Work out the finished part from the listing and answer in its coordinate system (mm). Face numbers are marked on the shaded views. A direction names the side the tool comes from. Give positions to 0.01 mm unless a question says otherwise; leave off trailing zeros. Loops run counter-clockwise (first coordinate to the right, second up) from the corner with the lowest first, then second, coordinate; pieces in that order, holes last. Notation, with made-up numbers: M 13.5,16.25 L 35.5,16.25 A11 cw 35.5,31.25 Z; hole C 83.5,-24 d10. An arc over 180 degrees is marked long. Write item = value, one per line. Start each with the question number.
1. Section B-B on z = 1.5 is taken. Determine the outline of the cut face in (x, y), plus the area to 3 significant figures.
2. Flat-ended cylindrical pins translate along their axes: pin 1 Ø6 at (x, z) = (9, 12) entering from +Y; pin 2 Ø4 at (x, y) = (0, -26.5) entering from -Z; pin 3 Ø5 at (y, z) = (18, 7) entering from -X; pin 4 Ø6 at (x, z) = (13, 8) entering from -Y. Find the tip coordinate at first contact, or state that the pin passes through.
3. For the marked faces 5, 6 and 7, determine the directions among +Z, -Z, +X, -X, +Y, -Y from which every point of the face is accessible in a straight line to the end or side of a thin tool.
4. Section C-C on y = -4 is taken. Determine the outline of the cut face in (x, z).
5. Section A-A on x = 0 is taken. Determine the outline of the cut face in (y, z), plus the area to 3 significant figures.
6. Section D-D on z = 9.5 is taken. Determine the outline of the cut face in (x, y), plus the area to 3 significant figures.
7. Consider L1, parallel to Y at x = 0, z = 4.25; L2, parallel to Z at x = 13, y = -1; L3, parallel to X at y = -26.5, z = 3.75. Determine where each line is inside the solid, lowest interval first. Write a range as [from, to].
8. The mould has two halves that part along Y. Classify the marked faces 1, 2, 3 and 4: released by +Y, released by -Y, zero draft, split by the parting line, or undercut.
```python
from build123d import *

# Parameters (mm, degrees)
SKETCH_1_R          = 21
EXTRUDE_2_DEPTH     = 6.5
EXTRUDE_4_DEPTH     = 6.5
SKETCH_3_R          = 9.5
SKETCH_3_R_2        = 3.5
CUT_EXTRUDE_1_DEPTH = 41.068691019


with BuildPart() as part:
    # 草图1 → 凸台-拉伸2 (new body)
    with BuildSketch(Plane.XY):
        with Locations(Location((0, 0, 0), (0, 0, 180))):
            Circle(SKETCH_1_R)
    extrude(amount=EXTRUDE_2_DEPTH)

    # 草图2 → 凸台-拉伸4 (add)
    with BuildSketch(Plane.XY):
        with BuildLine():
            Line((-7, -26.5), (-7, 26.5))
            ThreePointArc((-7, 26.5), (0, 33.5), (7, 26.5))
            Line((7, 26.5), (7, -26.5))
            ThreePointArc((7, -26.5), (0, -33.5), (-7, -26.5))
        make_face()
    extrude(amount=EXTRUDE_4_DEPTH)

    # 草图3 → 切除-拉伸1 (cut, through all)
    with BuildSketch(Plane.XY):
        with Locations(Location((0, 0, 0), (0, 0, 180))):
            Circle(SKETCH_3_R)
        with Locations(Location((0, -26.5, 0), (0, 0, 180))):
            Circle(SKETCH_3_R_2)
        with Locations(Location((0, 26.5, 0), (0, 0, 180))):
            Circle(SKETCH_3_R_2)
    extrude(amount=CUT_EXTRUDE_1_DEPTH, mode=Mode.SUBTRACT)

    # 草图4 → 旋转1 (revolve)
    with BuildSketch(Plane(origin=(0, 0, 0), x_dir=(0, 0, -1), z_dir=(1, 0, 0)), mode=Mode.PRIVATE) as revolve_1_sk:
        Polygon((0, 9.5), (0, 17), (-13, 17), (-13, 11), (-18.5, 11), (-18.5, 7.5), (-13, 7.5), (-13, 9.5), align=None)
    revolve(revolve_1_sk.sketch.rotate(Axis((0, 0, 23.5), (0, 0, -1)), 90), axis=Axis((0, 0, 23.5), (0, 0, -1)))


solid = part.part
```
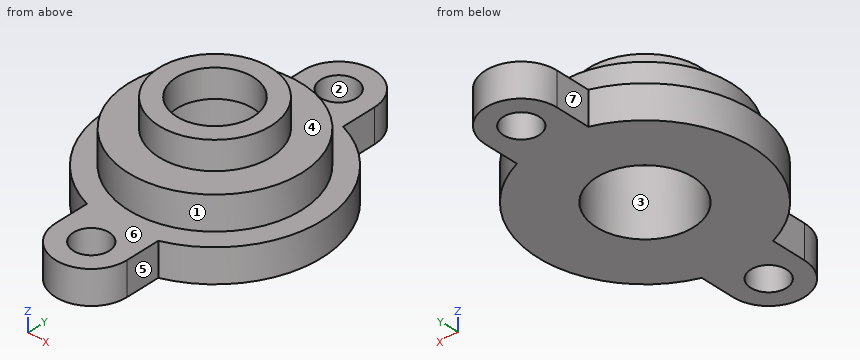
Verdict:
q1.outline = M -7,-26.5 A7 ccw 7,-26.5 L 7,-19.8 A21 ccw 7,19.8 L 7,26.5 A7 ccw -7,26.5 L -7,19.8 A21 ccw -7,-19.8 Z; hole C 0,0 d19; hole C 0,-26.5 d7; hole C 0,26.5 d7
q1.area = 1,340 mm2
q2.pin_1 = 15.91
q2.pin_2 = through
q2.pin_3 = -14.11
q2.pin_4 = -18.24
q3.face_5 = +Z, -Z, +X, -Y
q3.face_6 = +Z
q3.face_7 = +Z, -Z, -X, +Y
q4.outline = M -20.62,0 L -8.62,0 L -8.62,13 L -6.34,13 L -6.34,18.5 L -10.25,18.5 L -10.25,13 L -16.52,13 L -16.52,6.5 L -20.62,6.5 Z; M 6.34,13 L 8.62,13 L 8.62,0 L 20.62,0 L 20.62,6.5 L 16.52,6.5 L 16.52,13 L 10.25,13 L 10.25,18.5 L 6.34,18.5 Z
q5.outline = M -33.5,0 L -30,0 L -30,6.5 L -33.5,6.5 Z; M -23,0 L -9.5,0 L -9.5,13 L -7.5,13 L -7.5,18.5 L -11,18.5 L -11,13 L -17,13 L -17,6.5 L -23,6.5 Z; M 7.5,13 L 9.5,13 L 9.5,0 L 23,0 L 23,6.5 L 17,6.5 L 17,13 L 11,13 L 11,18.5 L 7.5,18.5 Z; M 30,0 L 33.5,0 L 33.5,6.5 L 30,6.5 Z
q5.area = 357 mm2
q6.outline = C 0,0 d34; hole C 0,0 d19
q6.area = 624 mm2
q7.L1 = [-33.5, -30], [-23, -9.5], [9.5, 23], [30, 33.5]
q7.L2 = [0, 13]
q7.L3 = [-7, -3.5], [3.5, 7]
q8.face_1 = split by the parting line
q8.face_2 = undercut
q8.face_3 = undercut
q8.face_4 = zero draft
